Autodesk Inventor part; units mm, degrees
ref_plane "РабПлоскость1" through (0, 30, 0) normal (0, 1, 0) x (-1, 0, 0)
ref_plane "YZ Plane" through (0, 0, 0) normal (1, 0, 0) x (0, 1, 0)
ref_plane "XY Plane" through (0, 0, 0) normal (0, 0, 1) x (1, 0, 0)
sketch "Эскиз1" plane through (0, 0, 0) normal (0, 0, 1) x (1, 0, 0)
  line L0 (0, 0) -> (20, 0)
  line L1 (20, 0) -> (20, 30)
  line L2 (20, 30) -> (0, 30)
  line L3 (0, 30) -> (0, 0)
  dimension "d0" = 20
  dimension "d1" = 30
revolve "Вращение1" add sketch "Эскиз1" angle 360 about axis through (0, 0, 0) along (1, 0, 0)
sketch "Эскиз2" plane through (0, 0, 0) normal (-1, 0, 0) x (0, 0, 1)
  circle A0 centre (0, 0) radius 26
  dimension "d3" = 52
extrude "Выдавливание1" cut sketch "Эскиз2" against normal blind 16
sketch "Эскиз3" plane through (0, 0, 0) normal (-1, 0, 0) x (0, 0, 1)
  line L0 (28, -30) -> (-28, -30)
  line L1 (-28, -30) -> (-28, 30)
  line L2 (-28, 30) -> (28, 30)
  line L3 (28, 30) -> (28, -30)
  circle A0 centre (0, 0) radius 30 construction
  point P0 (0, 30)
  dimension "d6" = 56
extrude "Выдавливание2" cut sketch "Эскиз3" against normal blind 20 keep common part
ref_plane "РабПлоскость1" through (0, 30, 0) normal (0, 1, 0) x (-1, 0, 0)
sketch "Эскиз4" plane through (0, 30, 0) normal (0, 1, 0) x (-1, 0, 0)
  line L0 (-20, 28) -> (0, 28) construction
  line L1 (0, -28) -> (-20, -28) construction
  line L2 (0, -28) -> (0, 28) construction
  line L3 (-20, 28) -> (0, 28)
  line L4 (-20, -28) -> (-20, 28) construction
  line L5 (0, 28) -> (0, -28)
  line L6 (0, 28) -> (-9.8743, -28)
  line L7 (0, -28) -> (-20, -28)
  line L8 (0, -28) -> (-9.8743, -28)
  line L9 (0, -28) -> (0, 28)
  point P0 (0, 0)
  dimension "d10" = 10
extrude "Выдавливание3" cut sketch "Эскиз4" against normal blind 60
properties part number "711123"
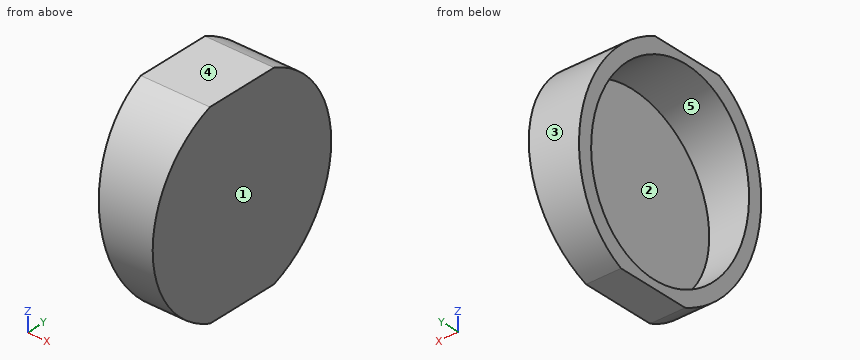
Geometry: final body of the model. Coordinates: model frame, mm. Face numbers are marked on the shaded views. A direction names the side the tool comes from. Round coordinates to 2 decimals unless told otherwise and drop trailing zeros. Loops run counter-clockwise (first coordinate to the right, second up) from the corner with the lowest first, then second, coordinate; pieces in that order, holes last.
Q1. Section D-D on x = 7.75. Return loops of the section in (y, z), plus the area to 3 significant figures.
Q2. Material intervals for L1, parallel to Y at x = 8.75, z = 0; L2, parallel to Z at x = 12.25, y = 0; L3, parallel to X at y = 16.5, z = 4, sorted ascending.
Q3. Pin query (flat end, axial travel): P1, Ø10, axis at x = 2, z = 12.5, coming from the +Y side; P2, Ø3, axis at y = 17.5, z = -9.5, coming from the -X side; P3, Ø2, axis at x = 4.5, y = -9.5, coming from the -Z side. Return the tip coordinate at first contact, or that it passes through.
Q4. Section C-C on z = 10. Return loops of the section in (x, y).
Q5. Section A-A on x = 12.75. Return loops of the section in (y, z), plus the area to 3 significant figures.
Q6. Section B-B on y = 0. Return loops of the section in (x, z), plus the area to 3 significant figures.
Q7. Access query for the marked faces 1 and 2. Directions: +Z, -Z, +X, -X, +Y, -Y. A direction counts if a zero-diameter tool reaches every point of the face in a straight line with its end or side. Return the directions, or none.
Q8. Pull-direction query (Y, two-part tool) for the marked faces 3, 4 and 5; classes: released by +Y, released by -Y, zero draft, split by the parting line, or undercut.
Evaluation:
1. outline: (-25.41, -15.95) - (-20.53, -15.95) arc R26 cw (long way) to (20.53, -15.95) - (25.41, -15.95) arc R30 ccw to (10.77, 28) - (-10.77, 28) arc R30 ccw to start
1. area: 459 mm2
2. L1: y = -30 to -26, 26 to 30
2. L2: z = -28 to -26, 26 to 28
2. L3: x = 16 to 20
3. P1: stops at y = 28.98
3. P2: stops at x = 16
3. P3: stops at z = 23.79
4. outline: (3.17, -28.28) - (20, -28.28) - (20, 28.28) - (3.17, 28.28) - (3.17, 24) - (16, 24) - (16, -24) - (3.17, -24) - close
5. outline: (-10.77, -28) - (10.77, -28) arc R30 ccw to (10.77, 28) - (-10.77, 28) arc R30 ccw to start; hole circle Ø52 at (0, 0)
5. area: 646 mm2
6. outline: (0, 28) - (0.35, 26) - (16, 26) - (16, -26) - (9.52, -26) - (9.87, -28) - (20, -28) - (20, 28) - close
6. area: 268 mm2
7. face 1: +Z, -Z, +X, +Y, -Y
7. face 2: -X
8. face 3: released by +Y
8. face 4: zero draft
8. face 5: undercut
